```python
from build123d import *

# Parameters (mm, degrees)
F1_DEPTH = 40
F2_SIZE  = 2.5
F3_W     = 102.5
F3_H     = 35
F3_H_2   = 2.5
F4_DEPTH = 459
F6_DEPTH = 20
F7_SIZE  = 2.5
F8_R     = 1.75


with BuildPart() as f1:
    # F0 (on Top) → F1 (new body)
    with BuildSketch(Plane.XY):
        with BuildLine():
            Line((-446.5, 0), (-12.5, 0))
            ThreePointArc((-12.5, 0), (-3.6611652352, 3.6611652352), (0, 12.5))
            Line((0, 12.5), (0, 584.5))
            ThreePointArc((0, 584.5), (-3.6611652352, 593.3388347648), (-12.5, 597))
            Line((-12.5, 597), (-446.5, 597))
            ThreePointArc((-446.5, 597), (-455.3388347648, 593.3388347648), (-459, 584.5))
            Line((-459, 584.5), (-459, 12.5))
            ThreePointArc((-459, 12.5), (-455.3388347648, 3.6611652352), (-446.5, 0))
        make_face()
    extrude(amount=F1_DEPTH)

    # F2
    f2_edges = [f1.edges().sort_by_distance(p)[0] for p in [
        (-229.5, 0, 40),
        (-3.661165, 3.661165, 40),
        (0, 298.5, 40),
        (-3.661165, 593.338835, 40),
        (-229.5, 597, 40),
        (-455.338835, 593.338835, 40),
        (-459, 298.5, 40),
        (-455.338835, 3.661165, 40),
        (-229.5, 0, 0),
        (-3.661165, 3.661165, 0),
        (0, 298.5, 0),
        (-3.661165, 593.338835, 0),
        (-229.5, 597, 0),
        (-455.338835, 593.338835, 0),
        (-459, 298.5, 0),
        (-455.338835, 3.661165, 0),
    ]]
    chamfer(f2_edges, length=F2_SIZE)

    # F3 (on face) → F4 (join)
    with BuildSketch(Plane(origin=(-459, 0, 0), x_dir=(0, -1, 0), z_dir=(-1, 0, 0))):
        with Locations((-470.75, 20)):
            Rectangle(F3_W, F3_H)
        with Locations((-470.75, 38.75)):
            Rectangle(F3_W, F3_H_2)
        with Locations((-470.75, 1.25)):
            Rectangle(F3_W, F3_H_2)
    extrude(amount=-F4_DEPTH)

    # F5 (on face) → F6 (cut)
    with BuildSketch(Plane.XY.offset(40)):
        with BuildLine():
            Line((-165.5, 572), (-293.5, 572))
            ThreePointArc((-293.5, 572), (-302.3388347648, 568.3388347648), (-306, 559.5))
            Line((-306, 559.5), (-306, 37.5))
            ThreePointArc((-306, 37.5), (-302.3388347648, 28.6611652352), (-293.5, 25))
            Line((-293.5, 25), (-165.5, 25))
            ThreePointArc((-165.5, 25), (-156.6611652352, 28.6611652352), (-153, 37.5))
            Line((-153, 37.5), (-153, 559.5))
            ThreePointArc((-153, 559.5), (-156.6611652352, 568.3388347648), (-165.5, 572))
        make_face()
    extrude(amount=-F6_DEPTH, mode=Mode.SUBTRACT)

    # F7
    f7_edges = [f1.edges().sort_by_distance(p)[0] for p in [
        (-306, 298.5, 40),
        (-229.5, 572, 20),
    ]]
    chamfer(f7_edges, length=F7_SIZE)

    # F8
    f8_edges = [f1.edges().sort_by_distance(p)[0] for p in [
        (-1.25, 419.5, 38.75),
        (-1.25, 522, 38.75),
        (-1.25, 419.5, 1.25),
        (-1.25, 522, 1.25),
        (-457.75, 522, 38.75),
        (-457.75, 419.5, 38.75),
        (-457.75, 522, 1.25),
        (-457.75, 419.5, 1.25),
    ]]
    fillet(f8_edges, radius=F8_R)


solid = f1.part
```
Design review of the part built by this model. Coordinates are the model's own, in mm. A direction names the side the tool comes from. Coordinates: 2 decimals unless noted, no trailing zeros. Loops run counter-clockwise (first coordinate to the right, second up) from the corner with the lowest first, then second, coordinate; pieces in that order, holes last. Notation, with made-up numbers: (47, -32.75) -> (89, -32.75) arc R8 cw to (89, -28.75) -> close; hole circle Ø6 at (32, 81.25). An arc over 180 degrees is marked (long way). Answer as a JSON object with one key per item and string values.
Q1. To check wall thickness, follow L1, parallel to Y at x = -188.5, z = 34; L2, parallel to Y at x = -164, z = 27.5; L3, parallel to X at y = 88.5, z = 30. State the ranges of each line that lie inside material, in increasing order.
Answer block:
{"L1": "y = 0 to 25, 572 to 597", "L2": "y = 0 to 25.09, 571.91 to 597", "L3": "x = -459 to -306, -153 to 0"}
Q2. The part is to be moulded in two halves that separate along Y. For faces 3 (the conical face through (-158.03, 29.87, 20.68)), 4 (the conical face through (-5.03, 4.87, 39.32)), 5 (the flat face through (-233, 303, 0)), say which applies: +Y half, -Y half, draft (parallel to the pull), parting line (faces both ways), or undercut.
Answer block:
{"face 3": "undercut", "face 4": "-Y half", "face 5": "draft"}
Q3. Tool access review of faces 1 (the cylindrical face through (-302.435, 28.759, 30.105)), 2 (the conical face through (-4.87, 591.97, 39.32)): name each direction out of +Z, -Z, +X, -X, +Y, -Y from which nothing blocks a thin tool from reaching the whole face with its end or side.
Answer block:
{"face 1": "+Z", "face 2": "+Z, +X, +Y"}
Q4. Take a section at B-B on x = -272. Give the boundary of the cut face in (y, z), plus the area to 3 significant figures.
Answer block:
{"outline": "(0, 2.5) -> (2.5, 0) -> (594.5, 0) -> (597, 2.5) -> (597, 37.5) -> (594.5, 40) -> (574.5, 40) -> (572, 37.5) -> (572, 22.5) -> (569.5, 20) -> (27.5, 20) -> (25, 22.5) -> (25, 37.5) -> (22.5, 40) -> (2.5, 40) -> (0, 37.5) -> close", "area": "12,900 mm^2"}
Q5. Take a section at C-C on y = 370. Give the boundary of the cut face in (x, z).
Answer block:
{"outline": "(-459, 2.5) -> (-456.5, 0) -> (-2.5, 0) -> (0, 2.5) -> (0, 37.5) -> (-2.5, 40) -> (-150.5, 40) -> (-153, 37.5) -> (-153, 22.5) -> (-155.5, 20) -> (-303.5, 20) -> (-306, 22.5) -> (-306, 37.5) -> (-308.5, 40) -> (-456.5, 40) -> (-459, 37.5) -> close"}
Q6. Take a section at A-A on y = 433.5. Give the boundary of the cut face in (x, z), plus the area to 3 significant figures.
Answer block:
{"outline": "(-459, 0) -> (0, 0) -> (0, 40) -> (-150.5, 40) -> (-153, 37.5) -> (-153, 22.5) -> (-155.5, 20) -> (-303.5, 20) -> (-306, 22.5) -> (-306, 37.5) -> (-308.5, 40) -> (-459, 40) -> close", "area": "15,300 mm^2"}
Q7. Clearance check with flat-ended pins moving along their axes: pin 1 Ø5 at (y, z) = (418.5, 36) entering from +X; pin 2 Ø3 at (x, y) = (-227, 85.5) entering from +Z. State where each tip first meets the part, or that it passes through.
Answer block:
{"pin 1": "stops at x = 0", "pin 2": "stops at z = 20"}
